Build history of the part. All positions in model axes, mm. Coordinates: 2 decimals unless noted, no trailing zeros. Write each loop counter-clockwise with the first axis right and the second up, starting at its lowest first coordinate (ties: lowest second). Pieces come first, ordered by that corner, then holes.
```python
from build123d import *

# Parameters (mm, degrees)
SKETCH_1_R                   = 5
EXTRUDE_1_DEPTH              = 12
HOLE_WIZARD_M4_1_D           = 3.3
HOLE_WIZARD_M4_1_CSINK_D     = 4.05
HOLE_WIZARD_M4_1_CSINK_ANGLE = 90
SKETCH_7_R                   = 5
CUT_EXTRUDE_1_DEPTH          = 2


with BuildPart() as part:
    # 草图1 → 凸台-拉伸1 (new body)
    with BuildSketch(Plane(origin=(0, 0, 0), x_dir=(1, 0, 0), z_dir=(0, 1, 0))):
        with Locations(Location((0, 0, 0), (0, 0, 270))):
            Circle(SKETCH_1_R)
    extrude(amount=EXTRUDE_1_DEPTH)

    # M4 螺纹孔1 (through all)
    with Locations(Plane.XZ):
        with Locations((0, 0)):
            CounterSinkHole(HOLE_WIZARD_M4_1_D / 2, HOLE_WIZARD_M4_1_CSINK_D / 2, counter_sink_angle=HOLE_WIZARD_M4_1_CSINK_ANGLE)

    # 草图7 → 切除-拉伸1 (cut)
    with BuildSketch(Plane.XZ):
        with Locations(Location((0, 0, 0), (0, 0, 270))):
            Circle(SKETCH_7_R)
    extrude(amount=-CUT_EXTRUDE_1_DEPTH, mode=Mode.SUBTRACT)


solid = part.part
```
1. Saw through at A-A on z = 0. List the corners of the cut face in (x, y).
Computed values:
outline: (-5, 2) - (-1.65, 2) - (-1.65, 12) - (-5, 12) - close; (1.65, 2) - (5, 2) - (5, 12) - (1.65, 12) - close
2. Saw through at B-B on x = 0. List the corners of the cut face in (y, z), plus the area to 3 significant figures.
Computed values:
outline: (2, -5) - (12, -5) - (12, -1.65) - (2, -1.65) - close; (2, 1.65) - (12, 1.65) - (12, 5) - (2, 5) - close
area: 67.0 mm2
3. Mould opens along X. For faces 1 (the face through (1.216, 7.07, 1.115)), 2 (the face through (0, 2, -2)), 3 (the face through (-4.88, 6.93, -1.08)) say: +X half, -X half, draft (parallel to the pull), parting line (faces both ways), or undercut.
Computed values:
face 1: undercut
face 2: draft
face 3: parting line
4. Flat gauge pins, fed straight in: pin 1 (2 mm diameter, centred on y = 7.5, z = 4, fed in from -X); pin 2 (6 mm diameter, centred on x = 0.5, z = 1, fed in from +Y). Where does each tip first touch, or does it go through?
Computed values:
pin 1: stops at x = -4
pin 2: stops at y = 12
5. Probe line 1 along Z through (x, y) = (0.25, 11.25); line 2 along X through (y, z) = (6.5, 0.5); line 3 along Z through (x, y) = (3.25, 11.75). List the from-to ranges inside material, lowest first.
Computed values:
line 1: z = -4.99 to -1.63, 1.63 to 4.99
line 2: x = -4.97 to -1.57, 1.57 to 4.97
line 3: z = -3.8 to 3.8
6. Saw through at C-C on y = 10.25. List the corners of the cut face in (x, z).
Computed values:
outline: circle Ø10 at (0, 0); hole circle Ø3.3 at (0, 0)
7. Saw through at D-D on z = 3. List the corners of the cut face in (x, y).
Computed values:
outline: (-4, 2) - (4, 2) - (4, 12) - (-4, 12) - close
